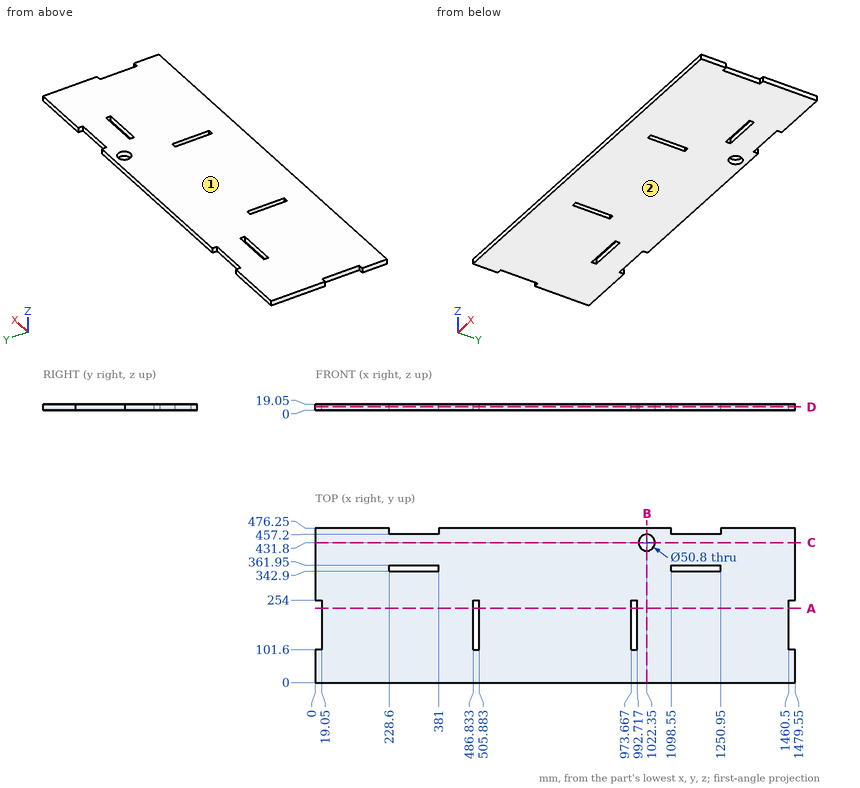
Study the drawing (mm; zero at the part's minimum x, y, z) and answer. Give positions to 0.01 mm unless a question says otherwise; leave off trailing zeros. Loops run counter-clockwise (first coordinate to the right, second up) from the corner with the lowest first, then second, coordinate; pieces in that order, holes last. Notation, with made-up numbers: (27, -28.5) - (39, -28.5) arc R31 ccw to (39, 4.5) - close; hole circle Ø8 at (11.25, 52). An arc over 180 degrees is marked (long way). Return JSON: item names as keys, results as strings. Group by question number.
1. Find section B-B (x = 1022.35). Write down the section's boundary in (y, z).
2. Find section C-C (y = 431.8). Write down the section's boundary in (x, z), then the cut area to 3 significant figures.
3. Determine the mould class of the marked faces 1 and 2 for opening direction Z: pulls with the +Z half, pulls with the -Z half, needs draft (parallel to the pull), parting line crosses it, or undercut.
4. Find section D-D (z = 10). State how many separate pieces and enclosed holes the cut face has, then the cut area to 3 significant figures.
5. Given pin 1 Ø9.5 at (x, z) = (323, 9.5) entering from +Y; pin 2 Ø4 at (y, z) = (92, 11) entering from -X; pin 3 Ø9.5 at (y, z) = (184.5, 6.5) entering from +X, each flat-ended and moving along its own axis, determine where each tip first touches the part or whether it passes through.
6. Find section A-A (y = 229). Write down the section's boundary in (x, z).
7. Straight lines are drawn through the part: line 1 (Y direction, x = 1022.35, z = 10); line 2 (X direction, y = 415.5, z = 16.5). For each, find the intervals that lie inside material, in ascending order. Write a range as [from, to].
Verdict:
{
 "1": {"outline": "(0, 0) - (406.4, 0) - (406.4, 19.05) - (0, 19.05) - close; (457.2, 0) - (476.25, 0) - (476.25, 19.05) - (457.2, 19.05) - close"},
 "2": {"outline": "(0, 0) - (996.95, 0) - (996.95, 19.05) - (0, 19.05) - close; (1047.75, 0) - (1479.55, 0) - (1479.55, 19.05) - (1047.75, 19.05) - close", "area": "27,200 mm^2"},
 "3": {"face 1": "pulls with the +Z half", "face 2": "pulls with the -Z half"},
 "4": {"separate pieces": "1", "enclosed holes": "5", "area": "679,000 mm^2"},
 "5": {"pin 1": "stops at y = 457.2", "pin 2": "stops at x = 0", "pin 3": "stops at x = 1460.5"},
 "6": {"outline": "(19.05, 0) - (486.83, 0) - (486.83, 19.05) - (19.05, 19.05) - close; (505.88, 0) - (973.67, 0) - (973.67, 19.05) - (505.88, 19.05) - close; (992.72, 0) - (1460.5, 0) - (1460.5, 19.05) - (992.72, 19.05) - close"},
 "7": {"line 1": "y = [0, 406.4], [457.2, 476.25]", "line 2": "x = [0, 1002.87], [1041.83, 1479.55]"}
}
